Drawing for the job (mm, zero at the part's lowest x, y, z). Round coordinates to 2 decimals unless told otherwise and drop trailing zeros. Order: outer loops, then holes, each group sorted by start corner. A loop starts at its lowest first (then second) coordinate and runs counter-clockwise, first axis right, second up. Notation, with made-up numbers: (2, -19) - (52, -19) arc R15 ccw to (52, -11) - close; hole circle Ø5 at (37, 76.25). An arc over 180 degrees is marked (long way). Answer as a JSON object with one key per item and string values.
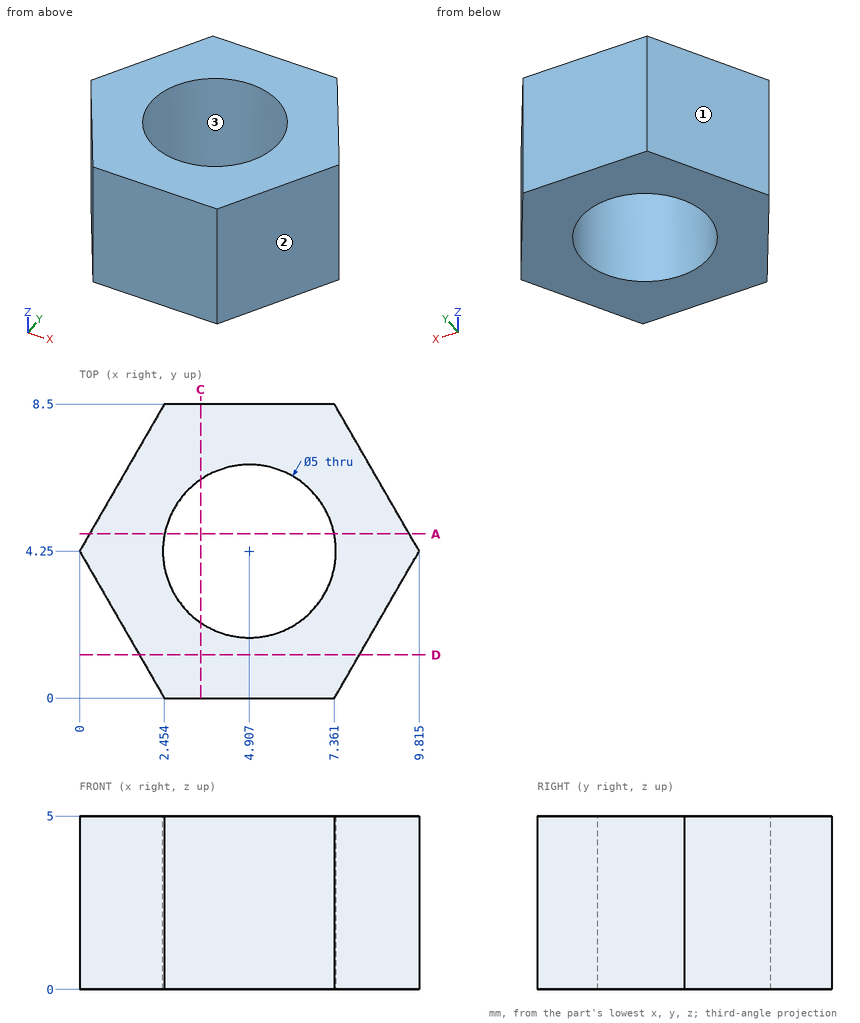
Item 1: Cut at C-C (x = 3.5). Write the cut outline in (y, z).
Taken from the geometry:
{"outline": "(0, 0) - (2.18, 0) - (2.18, 5) - (0, 5) - close; (6.32, 0) - (8.5, 0) - (8.5, 5) - (6.32, 5) - close"}
Item 2: Drop flat-ended pins along their axis: P1, Ø4, axis at x = 2, y = 5.5, coming from the -Z side; P2, Ø2, axis at y = 7.5, z = 2.5, coming from the -X side; P3, Ø2, axis at x = 8.5, z = 1, coming from the +Y side; P4, Ø1, axis at y = 3, z = 0.5, coming from the +X side. Give the stop position or say it passes through.
Taken from the geometry:
{"P1": "z = 0", "P2": "x = 1.3", "P3": "y = 8.26", "P4": "x = 9.38"}
Item 3: Cut at D-D (y = 1.25). Write the cut outline in (x, z).
Taken from the geometry:
{"outline": "(1.73, 0) - (8.08, 0) - (8.08, 5) - (1.73, 5) - close"}
Item 4: Probe L1, parallel to Y at x = 5, z = 4.4; L2, parallel to X at y = 2.5, z = 1.65 (1 decimal); L3, parallel to Y at x = 3.75, z = 0.4 (1 decimal). List the from-to ranges inside material, lowest first. Write a range as from..to.
Taken from the geometry:
{"L1": "0..1.75, 6.75..8.5", "L2": "1..3.1, 6.7..8.8", "L3": "0..2, 6.5..8.5"}
Item 5: Cut at A-A (y = 4.75). Write the cut outline in (x, z), plus the area to 3 significant figures.
Taken from the geometry:
{"outline": "(0.29, 0) - (2.46, 0) - (2.46, 5) - (0.29, 5) - close; (7.36, 0) - (9.53, 0) - (9.53, 5) - (7.36, 5) - close", "area": "21.7 mm2"}
Item 6: Two-plate mould, pull along Y, no slides. Class the marked faces 1, 2 and 3: pulls with the +Y half, pulls with the -Y half, needs draft (parallel to the pull), parting line crosses it, or undercut.
Taken from the geometry:
{"face 1": "pulls with the +Y half", "face 2": "pulls with the -Y half", "face 3": "undercut"}
